Autodesk Inventor part; units mm, degrees
ref_plane "YZ Plane" through (0, 0, 0) normal (1, 0, 0) x (0, 1, 0)
ref_plane "XZ Plane" through (0, 0, 0) normal (0, 1, 0) x (-1, 0, 0)
ref_plane "XY Plane" through (0, 0, 0) normal (0, 0, 1) x (1, 0, 0)
sketch "Sketch2" plane through (0, 0, 0) normal (0, 0, 1) x (1, 0, 0)
  line L0 (0, 2.45) -> (0, -2.45)
  line L1 (0, 2.45) -> (30, 2.45)
  line L2 (30, 2.45) -> (30, 29.95)
  line L3 (30, 29.95) -> (80, 29.95)
  line L4 (80, 29.95) -> (80, 25.05)
  line L5 (34.9, 3.55) -> (30.85, 3.55)
  line L6 (30.85, 3.55) -> (30.85, 2.45)
  line L7 (30.85, 2.45) -> (80, 2.45)
  line L8 (80, 2.45) -> (80, -2.45)
  line L9 (80, -2.45) -> (30.85, -2.45)
  line L10 (30.85, -2.45) -> (30.85, -3.55)
  line L11 (30.85, -3.55) -> (34.9, -3.55)
  line L12 (34.9, -3.55) -> (34.9, -25.05)
  line L13 (34.9, 3.55) -> (34.9, 25.05)
  line L14 (80, 25.05) -> (34.9, 25.05)
  line L15 (0, -2.45) -> (30, -2.45)
  line L16 (30, -2.45) -> (30, -29.95)
  line L17 (80, -25.05) -> (80, -29.95)
  line L18 (80, -29.95) -> (30, -29.95)
  line L19 (80, -25.05) -> (34.9, -25.05)
  line L20 (0, 2.45) -> (0, 3.55)
  line L21 (0, 3.55) -> (28.9, 3.55)
  line L22 (28.9, 3.55) -> (28.9, 31.05)
  line L23 (80, 29.95) -> (80, 31.05)
  line L24 (80, 31.05) -> (28.9, 31.05)
  line L25 (80, 25.05) -> (80, 23.95)
  line L26 (80, 23.95) -> (36, 23.95)
  line L27 (80, 2.45) -> (80, 3.55)
  line L28 (80, 3.55) -> (36, 3.55)
  line L29 (36, 3.55) -> (36, 23.95)
  line L30 (0, -2.45) -> (0, -3.55)
  line L31 (0, -3.55) -> (28.9, -3.55)
  line L32 (28.9, -3.55) -> (28.9, -31.05)
  line L33 (80, -2.45) -> (80, -3.55)
  line L34 (80, -3.55) -> (36, -3.55)
  line L35 (36, -3.55) -> (36, -23.95)
  line L36 (80, -25.05) -> (80, -23.95)
  line L37 (80, -23.95) -> (36, -23.95)
  line L38 (80, -29.95) -> (80, -31.05)
  line L39 (80, -31.05) -> (28.9, -31.05)
  line L40 (0, 3.55) -> (0, 4.55)
  line L41 (0, 4.55) -> (27.9, 4.55)
  line L42 (27.9, 4.55) -> (27.9, 32.05)
  line L43 (80, 3.55) -> (80, 4.55)
  line L44 (80, 4.55) -> (37, 4.55)
  line L45 (37, 4.55) -> (37, 22.95)
  line L46 (80, 23.95) -> (80, 22.95)
  line L47 (80, 22.95) -> (37, 22.95)
  line L48 (80, 31.05) -> (80, 32.05)
  line L49 (80, 32.05) -> (27.9, 32.05)
  line L50 (0, -3.55) -> (0, -4.55)
  line L51 (0, -4.55) -> (27.9, -4.55)
  line L52 (27.9, -4.55) -> (27.9, -32.05)
  line L53 (80, -31.05) -> (80, -32.05)
  line L54 (80, -32.05) -> (27.9, -32.05)
  line L55 (80, -23.95) -> (80, -22.95)
  line L56 (80, -22.95) -> (37, -22.95)
  line L57 (80, -3.55) -> (80, -4.55)
  line L58 (80, -4.55) -> (37, -4.55)
  line L59 (37, -4.55) -> (37, -22.95)
  line L60 (80, 22.95) -> (80, 4.55)
  line L61 (80, -4.55) -> (80, -22.95)
  line L62 (40, -15) -> (70, -15) construction
  line L63 (70, -15) -> (70, 15) construction
  line L64 (70, 15) -> (40, 15) construction
  line L65 (40, 15) -> (40, -15) construction
  line L66 (40, -15) -> (70, 15) construction
  line L67 (70, -15) -> (40, 15) construction
  line L68 (55, 0) -> (0, 0) construction
  circle A0 centre (70, 15) radius 1.6
  circle A1 centre (40, 15) radius 1.6
  circle A2 centre (70, -15) radius 1.6
  circle A3 centre (40, -15) radius 1.6
  dimension "d21" = 4.9
  dimension "d23" = 4.9
  dimension "d27" = 30
  dimension "d28" = 4.05
  dimension "d29" = 1.1
  dimension "d31" = 1.1
  dimension "d33" = 1.1
  dimension "d34" = 1.1
  dimension "d35" = 1.1
  dimension "d36" = 1.1
  dimension "d37" = 1.1
  dimension "d38" = 1.1
  dimension "d39" = 1
  dimension "d40" = 1
  dimension "d41" = 1
  dimension "d42" = 1
  dimension "d43" = 1
  dimension "d44" = 1
  dimension "d54" = 30
  dimension "d55" = 30
  dimension "d57" = 3.2
  dimension "d58" = 3.2
  dimension "d59" = 3.2
  dimension "d60" = 3.2
  dimension "d75" = 1.1
  dimension "d76" = 1
  dimension "d77" = 1.1
  dimension "d78" = 1
  dimension "d79" = 4.9
  dimension "d80" = 4.9
  dimension "d81" = 50.1
  dimension "d83" = 55
  dimension "d84" = 80
extrude "Extrusion1" add sketch "Sketch2" along normal blind 2 contours L1 L2 L3 L4 L14 L13 L5 L6 L7 L8 L9 L10 L11 L12 L19 L17 L18 L16 L15 L0
extrude "Extrusion2" add sketch "Sketch2" along normal blind 1 contours L1 L2 L3 L4 L14 L13 L5 L6 L7 L8 L9 L10 L11 L12 L19 L17 L18 L16 L15 L0 | L20 L21 L22 L24 L23 L3 L2 L1 | L15 L16 L18 L38 L39 L32 L31 L30 | L25 L26 L29 L28 L27 L7 L6 L5 L13 L14 | L19 L12 L11 L10 L9 L33 L34 L35 L37 L36
extrude "Extrusion3" add sketch "Sketch2" along normal blind 4 contours L40 L41 L42 L49 L48 L24 L22 L21 | L31 L32 L39 L53 L54 L52 L51 L50 | L46 L47 L45 L44 L43 L28 L29 L26 | L37 L35 L34 L57 L58 L59 L56 L55
extrude "Extrusion4" add sketch "Sketch2" along normal up to surface (4 mm away) contours L60 L44 L45 L47 | L56 L59 L58 L61
sketch "Sketch3" plane through (0, 0, 0) normal (0, 0, -1) x (-1, 0, 0)
  line L0 (-52.5, -2.5) -> (-57.5, -2.5)
  line L1 (-57.5, -2.5) -> (-57.5, 2.5)
  line L2 (-57.5, 2.5) -> (-52.5, 2.5)
  line L3 (-52.5, 2.5) -> (-52.5, -2.5)
  line L4 (-52.5, -2.5) -> (-57.5, 2.5) construction
  line L5 (-57.5, -2.5) -> (-52.5, 2.5) construction
  line L6 (-55, 0) -> (0, 0) construction
  line L7 (-80, -4.55) -> (-80, 4.55)
  line L8 (-49, -6) -> (-61, -6)
  line L9 (-61, -6) -> (-61, 6)
  line L10 (-61, 6) -> (-49, 6)
  line L11 (-49, 6) -> (-49, -6)
  line L12 (-49, -6) -> (-61, 6) construction
  line L13 (-61, -6) -> (-49, 6) construction
  dimension "d51" = 5
  dimension "d52" = 5
  dimension "d53" = 25
  dimension "d65" = 12
  dimension "d66" = 12
extrude "Extrusion5" cut sketch "Sketch3" against normal blind 2 contours L0 L1 L2 L3
extrude "Extrusion6" cut sketch "Sketch3" against normal blind 0.5
sketch "Sketch4" plane through (80, -2.45, 2) normal (1, 0, 0) x (0, 0, -1)
  line L0 (0, 27.5) -> (0, 32.4)
  line L1 (0, 32.4) -> (0.9, 32.4)
  line L2 (0.9, 32.4) -> (0.9, 27.5)
  line L3 (0.9, 27.5) -> (0, 27.5)
  line L4 (0, 27.5) -> (0, 32.4)
  line L5 (1, 27.5) -> (0, 27.5)
  line L6 (0, 0) -> (0, 4.9)
  line L7 (0, 4.9) -> (0.9, 4.9)
  line L8 (0.9, 4.9) -> (0.9, 0)
  line L9 (0.9, 0) -> (0, 0)
  line L10 (0, 0) -> (0, 4.9)
  line L11 (0.9, -22.6) -> (0, -22.6)
  line L12 (0.9, -22.6) -> (0.9, -27.5)
  line L13 (0.9, -27.5) -> (0, -27.5)
  line L14 (0, -27.5) -> (0, -22.6)
  line L15 (1, -27.5) -> (0, -27.5)
  line L16 (1, 0) -> (0, 0)
  line L17 (1, -22.6) -> (0, -22.6)
  line L18 (0, -27.5) -> (0, -22.6)
  point P0 (2, 2.45)
  dimension "d69" = 0.9
extrude "Extrusion7" add sketch "Sketch4" along normal blind 5
sketch "Sketch5" plane through (0, -2.45, 2) normal (-1, 0, 0) x (0, 0, 1)
  line L0 (0, 4.9) -> (-0.9, 4.9)
  line L1 (-0.9, 4.9) -> (-0.9, 0)
  line L2 (-0.9, 0) -> (0, 0)
  line L3 (0, 0) -> (0, 4.9)
  line L4 (0, 4.9) -> (0, 0)
  line L5 (-1, 0) -> (0, 0)
  line L6 (-1, 4.9) -> (0, 4.9)
  line L7 (-1, 6) -> (-1, 4.9)
  point P0 (-2, 2.45)
  dimension "d72" = 0.1
extrude "Extrusion8" add sketch "Sketch5" along normal blind 5
properties part number "bottomv6"
Input: part model. Units: mm. Frame: model coordinates. A direction names the side the tool comes from. Round coordinates to 2 decimals unless told otherwise and drop trailing zeros. Order: outer loops, then holes, each group sorted by start corner. A loop starts at its lowest first (then second) coordinate and runs counter-clockwise, first axis right, second up. Notation, with made-up numbers: (41.25, -17.5) - (95.25, -17.5) arc R20 cw to (95.25, 7.5) - close; hole circle Ø1 at (-36.5, 14). An arc over 180 degrees is marked (long way). Answer as a JSON object with one key per item and string values. Group by question number.
(1) Material intervals for probe 1 along Y at (x, z) = (76, 3.35); probe 2 along Y at (x, z) = (70, 2.7); probe 3 along Y at (x, z) = (70, 0.6), sorted ascending. Write a range as from..to.
(2) Cut plane D-D (x = 74). Return loops of the section in (y, z).
(3) Cut plane C-C (y = -0.5). Return loops of the section in (x, z).
(4) Cut plane A-A (z = 3). Return loops of the section in (x, y), then the cut area to 3 significant figures.
(5) Pin query (flat end, axial travel): P1, Ø1, axis at x = 7, z = 3, coming from the +Y side; P2, Ø6, axis at x = 54.5, y = -1, coming from the -Z side; P3, Ø3, axis at x = 19, y = -6.5, coming from the +Z side; P4, Ø2.5, axis at x = 82.5, y = -28, coming from the -Z side. Return the tip coordinate at first contact, or that it passes through.
(6) Cut plane B-B (y = -15). Return loops of the section in (x, z), then the cut area to 3 significant figures.
(7) Draft query along X for faces 4 (the face through (39.792, -16.586, 1.972)), 5 (the face through (14, -4.55, 2)), 6 (the face through (39.792, 13.414, 1.972)), 7 (the face through (80, 0.4, 0.6)). Return one class per face: released by +X, released by -X, zero draft, split by the parting line, or undercut.
(8) Reachability of faces 1 (the face through (55, -31.05, 2)), 2 (the face through (14, -3.55, 2)), 3 (the face through (40, -2, 2)) from +Z, -Z, +X, -X, +Y, -Y: full face, straight path, thin tool, end or side. Return the list, or none.
Here are the results:
{
 "1": {"probe 1": "y = -32.05..-31.05, -23.95..-3.55, 3.55..23.95, 31.05..32.05", "probe 2": "y = -32.05..-31.05, -23.95..-16.6, -13.4..-3.55, 3.55..13.4, 16.6..23.95, 31.05..32.05", "probe 3": "y = -32.05..-16.6, -13.4..13.4, 16.6..32.05"},
 "2": {"outline": "(-32.05, 0) - (32.05, 0) - (32.05, 4) - (31.05, 4) - (31.05, 1) - (29.95, 1) - (29.95, 2) - (25.05, 2) - (25.05, 1) - (23.95, 1) - (23.95, 4) - (3.55, 4) - (3.55, 1) - (2.45, 1) - (2.45, 2) - (-2.45, 2) - (-2.45, 1) - (-3.55, 1) - (-3.55, 4) - (-23.95, 4) - (-23.95, 1) - (-25.05, 1) - (-25.05, 2) - (-29.95, 2) - (-29.95, 1) - (-31.05, 1) - (-31.05, 4) - (-32.05, 4) - close"},
 "3": {"outline": "(-5, 1.1) - (0, 1.1) - (0, 0) - (49, 0) - (49, 0.5) - (52.5, 0.5) - (52.5, 2) - (-5, 2) - close; (57.5, 0.5) - (61, 0.5) - (61, 0) - (80, 0) - (80, 1.1) - (85, 1.1) - (85, 2) - (57.5, 2) - close"},
 "4": {"outline": "(0, -4.55) - (27.9, -4.55) - (27.9, -32.05) - (80, -32.05) - (80, -31.05) - (28.9, -31.05) - (28.9, -3.55) - (0, -3.55) - close; (0, 3.55) - (28.9, 3.55) - (28.9, 31.05) - (80, 31.05) - (80, 32.05) - (27.9, 32.05) - (27.9, 4.55) - (0, 4.55) - close; (36, -23.95) - (80, -23.95) - (80, -3.55) - (36, -3.55) - close; (36, 3.55) - (80, 3.55) - (80, 23.95) - (36, 23.95) - close; hole circle Ø3.2 at (40, -15); hole circle Ø3.2 at (40, 15); hole circle Ø3.2 at (70, -15); hole circle Ø3.2 at (70, 15)", "area": "1,980 mm^2"},
 "5": {"P1": "stops at y = 4.55", "P2": "stops at z = 0.5", "P3": "passes through", "P4": "stops at z = 1.1"},
 "6": {"outline": "(27.9, 0) - (38.4, 0) - (38.4, 4) - (36, 4) - (36, 1) - (34.9, 1) - (34.9, 2) - (30, 2) - (30, 1) - (28.9, 1) - (28.9, 4) - (27.9, 4) - close; (41.6, 0) - (68.4, 0) - (68.4, 4) - (41.6, 4) - close; (71.6, 0) - (80, 0) - (80, 4) - (71.6, 4) - close", "area": "166 mm^2"},
 "7": {"face 4": "undercut", "face 5": "zero draft", "face 6": "undercut", "face 7": "released by +X"},
 "8": {"face 1": "+Z, +X", "face 2": "+Z, -X", "face 3": "+Z"}
}
